Model file for the job. Use its own axes, mm. A direction names the side the tool comes from. Round coordinates to 2 decimals unless told otherwise and drop trailing zeros. Loops run counter-clockwise (first coordinate to the right, second up) from the corner with the lowest first, then second, coordinate; pieces in that order, holes last. Notation, with made-up numbers: M 27,60 L 52,60 A28 ccw 52,80 Z; hole C -34.5,-23.5 d8. An arc over 180 degrees is marked long. Answer in a Markdown table with one row per item.
from build123d import *

# Parameters (mm, degrees)
SKETCH1_R           = 25
BOSS_EXTRUDE1_DEPTH = 45
CHAMFER1_SIZE       = 5
CHAMFER1_SIZE2      = 1.819851171
SKETCH2_R           = 3
BOSS_EXTRUDE2_DEPTH = 22
BOSS_EXTRUDE3_START = 2
SKETCH3_R           = 3
BOSS_EXTRUDE3_DEPTH = 2
CIRPATTERN1_COUNT   = 4


with BuildPart() as part:
    # Sketch1 → Boss-Extrude1 (new body)
    with BuildSketch(Plane.XY):
        with Locations(Location((0, 0, 0), (0, 0, 180))):
            Circle(SKETCH1_R)
    extrude(amount=BOSS_EXTRUDE1_DEPTH)

    # Chamfer1
    chamfer1_edges = [part.edges().sort_by_distance(p)[0] for p in [
        (25, 0, 0),
        (25, 0, 45),
    ]]
    chamfer1_side = [part.faces().sort_by_distance(p)[0] for p in [
        (25, 0, 22.5),
    ]]
    chamfer(chamfer1_edges, length=CHAMFER1_SIZE, length2=CHAMFER1_SIZE2, reference=chamfer1_side[0])

    # Sketch2 → Boss-Extrude2 (add)
    with BuildSketch(Plane.XY.offset(45)):
        Circle(SKETCH2_R)
    extrude(amount=BOSS_EXTRUDE2_DEPTH)

    # Sketch3 → Boss-Extrude3 (add)
    with BuildSketch(Plane(origin=(0, 0, 0), x_dir=(-1, 0, 0), z_dir=(0, 0, -1)).offset(BOSS_EXTRUDE3_START)):
        with Locations(Location((0, 0, 0), (0, 0, 180))):
            Circle(SKETCH3_R)
    extrude(amount=-BOSS_EXTRUDE3_DEPTH)

    # Sketch5 → Tap Drill for M3x0.5 Tap1 (revolve, cut)
    with BuildSketch(Plane(origin=(0, 10, 0), x_dir=(0, 1, 0), z_dir=(1, 0, 0))):
        Polygon((0, 0), (0, 10.751075774), (1.25, 10), (1.25, 0), align=None)
    tap_drill_for_m3x0_5_tap1 = revolve(axis=Axis((0, 10, -6.35), (0, 0, 1)), mode=Mode.SUBTRACT)

    # CirPattern1: Tap Drill for M3x0.5 Tap1 ×4 about axis
    cirpattern1_axis = Axis((0, 0, 0), (0, 0, 1))
    for i in range(1, CIRPATTERN1_COUNT):
        add(tap_drill_for_m3x0_5_tap1.rotate(cirpattern1_axis, i * 360 / CIRPATTERN1_COUNT), mode=Mode.SUBTRACT)


solid = part.part
1. Saw through at B-B (z = 20). Write the cut outline in (x, y), and give its area (3 significant figures).
Verdict:
| item | result |
|---|---|
| outline | C 0,0 d50 |
| area | 1,960 mm² |
2. Mould opens along X. For faces 4 (the cylindrical face through (-23.846, -7.509, 22.255)), 5 (the flat face through (-5, 0, 0)), 6 (the conical face through (10.21, 0.07, 10.62)) say: +X half, -X half, draft (parallel to the pull), parting line (faces both ways), or undercut.
Verdict:
| item | result |
|---|---|
| face 4 | parting line |
| face 5 | draft |
| face 6 | undercut |
3. Tool access for faces 1 (the cylindrical face through (2.86, -0.9, -1.01)), 2 (the flat face through (0, 0, 67)), 3 (the cylindrical face through (-3, 0, 56)): list every direction of +Z, -Z, +X, -X, +Y, -Y with a clear straight run to the whole face (end or side of a thin tool).
Verdict:
| item | result |
|---|---|
| face 1 | -Z |
| face 2 | +Z, +X, -X, +Y, -Y |
| face 3 | +Z |
4. Wall check: probe 1 along Y at (x, z) = (10, 5); probe 2 along Y at (x, z) = (10, 4); probe 3 along Z at (x, y) = (-12.5, -0.5). Give the ranges that are in metal, low to high.
Verdict:
| item | result |
|---|---|
| probe 1 | y = -22.91 to -1.25, 1.25 to 22.91 |
| probe 2 | y = -22.52 to -1.25, 1.25 to 22.52 |
| probe 3 | z = 0 to 45 |
5. Pin check, flat tips, straight feed: pin 1 (3 mm diameter, centred on y = -18.5, z = 25.5, fed in from -X); pin 2 (12 mm diameter, centred on x = 10.5, z = 34.5, fed in from +Y); pin 3 (3 mm diameter, centred on x = 13, z = 34.5, fed in from -Y). Stop position of each tip, or through.
Verdict:
| item | result |
|---|---|
| pin 1 | stops at x = -18.33 |
| pin 2 | stops at y = 24.59 |
| pin 3 | stops at y = -22.2 |
6. Saw through at A-A (z = 8). Write the cut outline in (x, y).
Verdict:
| item | result |
|---|---|
| outline | C 0,0 d50; hole C -10,0 d2.5; hole C 0,-10 d2.5; hole C 0,10 d2.5; hole C 10,0 d2.5 |
7. Saw through at C-C (z = 52). Write the cut outline in (x, y).
Verdict:
| item | result |
|---|---|
| outline | C 0,0 d6 |
